```python
from build123d import *

# Parameters (mm, degrees)
SKETCH1_R               = 38.1
BOSS_EXTRUDE1_DEPTH     = 25.4
SKETCH2_R               = 38.1
SKETCH2_R_2             = 25.4
BOSS_EXTRUDE2_DEPTH     = 25.4
SKETCH3_R               = 38.1
BOSS_EXTRUDE3_DEPTH     = 25.4
SKETCH4_R               = 12.7
CUT_EXTRUDE1_DEPTH      = 77.2
FILLET1_R               = 2.54
SKETCH6_R               = 1.905
CUT_EXTRUDE2_DEPTH      = 39.1000001
CUT_EXTRUDE2_DEPTH_BACK = 39.1000001
SKETCH7_R               = 3.81
CUT_EXTRUDE3_DEPTH      = 25.4
SKETCH8_R               = 3.81
CUT_EXTRUDE4_DEPTH      = 25.4
CUT_EXTRUDE5_REACH      = 78.2
SKETCH9_W               = 50.8
SKETCH9_H               = 76.2
FILLET2_R               = 2.54
SKETCH10_R              = 3.175
CUT_EXTRUDE6_DEPTH      = 77.2
FILLET3_R               = 2.54


with BuildPart() as part:
    # Sketch1 → Boss-Extrude1 (new body)
    with BuildSketch(Plane(origin=(0, 0, 0), x_dir=(0, 0, -1), z_dir=(1, 0, 0))):
        Circle(SKETCH1_R)
    extrude(amount=BOSS_EXTRUDE1_DEPTH)

    # Sketch2 → Boss-Extrude2 (add)
    with BuildSketch(Plane(origin=(25.4, 0, 0), x_dir=(0, 0, -1), z_dir=(1, 0, 0))):
        Circle(SKETCH2_R)
        Circle(SKETCH2_R_2, mode=Mode.SUBTRACT)
    extrude(amount=BOSS_EXTRUDE2_DEPTH)

    # Sketch3 → Boss-Extrude3 (add)
    with BuildSketch(Plane(origin=(50.8, 0, 0), x_dir=(0, 0, -1), z_dir=(1, 0, 0))):
        Circle(SKETCH3_R)
    extrude(amount=BOSS_EXTRUDE3_DEPTH)

    # Sketch4 → Cut-Extrude1 (cut, through all)
    with BuildSketch(Plane(origin=(76.2, 0, 0), x_dir=(0, 0, -1), z_dir=(1, 0, 0))):
        Circle(SKETCH4_R)
    extrude(amount=-CUT_EXTRUDE1_DEPTH, mode=Mode.SUBTRACT)

    # Fillet1
    fillet1_edges = [part.edges().sort_by_distance(p)[0] for p in [
        (76.2, 0, 38.1),
        (0, 0, 38.1),
    ]]
    fillet(fillet1_edges, radius=FILLET1_R)

    # Sketch6 → Cut-Extrude2 (cut, two sides)
    with BuildSketch(Plane.XY) as cut_extrude2_sk:
        with Locations((30.48, 31.75)):
            Circle(SKETCH6_R)
        with Locations((45.72, 31.75)):
            Circle(SKETCH6_R)
        with Locations((30.48, -31.75)):
            Circle(SKETCH6_R)
        with Locations((45.72, -31.75)):
            Circle(SKETCH6_R)
    extrude(amount=CUT_EXTRUDE2_DEPTH, mode=Mode.SUBTRACT)
    extrude(cut_extrude2_sk.sketch, amount=-CUT_EXTRUDE2_DEPTH_BACK, mode=Mode.SUBTRACT)

    # Sketch7 → Cut-Extrude3 (cut)
    with BuildSketch(Plane.XY.offset(15.24)):
        with Locations((30.48, 31.75)):
            Circle(SKETCH7_R)
        with Locations((45.72, -31.75)):
            Circle(SKETCH7_R)
    extrude(amount=CUT_EXTRUDE3_DEPTH, mode=Mode.SUBTRACT)

    # Sketch8 → Cut-Extrude4 (cut)
    with BuildSketch(Plane.XY.offset(-15.24)):
        with Locations((45.72, 31.75)):
            Circle(SKETCH8_R)
        with Locations((30.48, -31.75)):
            Circle(SKETCH8_R)
    extrude(amount=-CUT_EXTRUDE4_DEPTH, mode=Mode.SUBTRACT)

    # Sketch9 → Cut-Extrude5 (cut, up to next)
    with BuildSketch(Plane.ZY, mode=Mode.PRIVATE) as cut_extrude5_sk1:
        with Locations((-25.4, 0)):
            Rectangle(SKETCH9_W, SKETCH9_H)
    cut_extrude5_tool1 = extrude(cut_extrude5_sk1.sketch, amount=-CUT_EXTRUDE5_REACH, mode=Mode.PRIVATE) & part.part
    add(cut_extrude5_tool1.solids().sort_by_distance((0, 0, -25.4))[0], mode=Mode.SUBTRACT)

    # Fillet2
    fillet2_edges = [part.edges().sort_by_distance(p)[0] for p in [
        (25.4, 0, 12.7),
        (50.8, 0, 12.7),
    ]]
    fillet(fillet2_edges, radius=FILLET2_R)

    # Sketch10 → Cut-Extrude6 (cut, through all)
    with BuildSketch(Plane(origin=(76.2, 0, 0), x_dir=(0, 0, -1), z_dir=(1, 0, 0))):
        with Locations((-31.75, 0)):
            Circle(SKETCH10_R)
    extrude(amount=-CUT_EXTRUDE6_DEPTH, mode=Mode.SUBTRACT)

    # Fillet3
    fillet3_edges = [part.edges().sort_by_distance(p)[0] for p in [
        (0, 0, 12.7),
        (76.2, 0, 12.7),
    ]]
    fillet(fillet3_edges, radius=FILLET3_R)


solid = part.part
```
CAD build for the part. Positions are in the model's coordinates, mm. A direction names the side the tool comes from. Coordinates: 2 decimals unless noted, no trailing zeros. Order: outer loops, then holes, each group sorted by start corner. A loop starts at its lowest first (then second) coordinate and runs counter-clockwise, first axis right, second up. Notation, with made-up numbers: (38, 28.25) - (44, 28.25) arc R19 ccw to (44, 47.25) - close; hole circle Ø5 at (10, 16). An arc over 180 degrees is marked (long way). Use a Markdown table: item, result. Add a question column.
(1) Flat gauge pins, fed straight in: pin 1 (5.5 mm diameter, centred on x = 45.5, y = -31, fed in from +Z); pin 2 (3 mm diameter, centred on x = 40, y = 9.5, fed in from -Z); pin 3 (6 mm diameter, centred on y = -20, z = 11.5, fed in from -X); pin 4 (1.5 mm diameter, centred on x = 26.5, z = 29.5, fed in from +Y). Where does each tip first touch, or does it go through?
(2) Pull direction Z, two halves, no side cores. Call faces 4 (the face through (30.23, -29.86, 11.68)), 5 (the face through (38.63, 0.14, 34.92)), 6 (the face through (37.922, 0.559, 25.394)): +Z half, -Z half, draft (parallel to the pull), parting line (faces both ways), or undercut.
(3) Saw through at A-A (y = 0). Give the cut face in (x, z) (3 decimals).
(4) Drill centre lines: line 1 along X through (y, z) = (-31.75, 6.5) (3 decimals); line 2 along X through (y, z) = (23, 3); line 3 along X through (y, z) = (-30.5, 11). Where is each one in solid material? Low to high. Write a range as [from, to].
(5) Which spindle directions (+Z, -Z, +X, -X, +Y, -Y) get a long thin tool onto all of the face, cutting with end or side? Do faces 1 (the face through (30.344, 27.942, 19.313)), 2 (the face through (50.8, 0, 16)), 3 (the face through (37.6, 0.84, 38.09)). Say none if no direction does.
(6) Saw through at D-D (y = 31.75). Count the separate pieces of the cut face and the enclosed holes in it, then the cut area to 3 significant figures.
(7) Saw through at C-C (x = 62). Give the cut face in (y, z) (3 decimals).
(8) Saw through at B-B (x = 30.48). Give the cut face in (y, z) (3 decimals), then the cut area to 3 significant figures.
Solved:
| question | item | result |
|---|---|---|
| 1 | pin 1 | stops at z = 15.24 |
| 1 | pin 2 | stops at z = 22.89 |
| 1 | pin 3 | stops at x = 0 |
| 1 | pin 4 | stops at y = 25 |
| 2 | face 4 | draft |
| 2 | face 5 | undercut |
| 2 | face 6 | -Z half |
| 3 | outline | (0, 15.24) arc R2.54 ccw to (2.54, 12.7) - (22.86, 12.7) arc R2.54 ccw to (25.4, 15.24) - (25.4, 25.4) - (50.8, 25.4) - (50.8, 15.24) arc R2.54 ccw to (53.34, 12.7) - (73.66, 12.7) arc R2.54 ccw to (76.2, 15.24) - (76.2, 28.575) - (0, 28.575) - close; (0, 34.925) - (76.2, 34.925) - (76.2, 35.56) arc R2.54 ccw to (73.66, 38.1) - (2.54, 38.1) arc R2.54 ccw to (0, 35.56) - close |
| 4 | line 1 | x = [0, 28.575], [32.385, 43.815], [47.625, 76.2] |
| 4 | line 2 | x = [0, 25.4], [50.8, 76.2] |
| 4 | line 3 | x = [0, 29.04], [31.92, 44.28], [47.16, 76.2] |
| 5 | face 1 | +Z |
| 5 | face 2 | -Z |
| 5 | face 3 | +Z, +X, -X |
| 6 | separate pieces | 3 |
| 6 | enclosed holes | 0 |
| 6 | area | 1,420 mm² |
| 7 | outline | (-38.1, 0) - (-12.7, 0) arc R12.7 cw to (12.7, 0) - (38.1, 0) arc R38.1 ccw to start; hole circle Ø6.35 at (0, 31.75) |
| 8 | outline | (-38.1, 0) - (-33.655, 0) - (-33.655, 17.859) arc R38.1 ccw to start; (-29.845, 0) - (-25.4, 0) arc R25.4 cw to (25.4, 0) - (29.845, 0) - (29.845, 15.24) - (27.94, 15.24) - (27.94, 25.903) arc R38.1 ccw to (-29.845, 23.683) - close; (33.655, 0) - (38.1, 0) arc R38.1 ccw to (34.919, 15.24) - (33.655, 15.24) - close; hole circle Ø6.35 at (0, 31.75) |
| 8 | area | 1,060 mm² |
